Input: part model. Units: mm. Frame: model coordinates. Coordinates: 2 decimals unless noted, no trailing zeros. Order: outer loops, then holes, each group sorted by start corner. A loop starts at its lowest first (then second) coordinate and runs counter-clockwise, first axis right, second up. Notation, with made-up numbers: (-6.5, -26) -> (45.5, -26) arc R6 cw to (45.5, -19) -> close; hole circle Ø9 at (74.5, 33). An arc over 180 degrees is marked (long way). One line per question, with ' | ' between items.
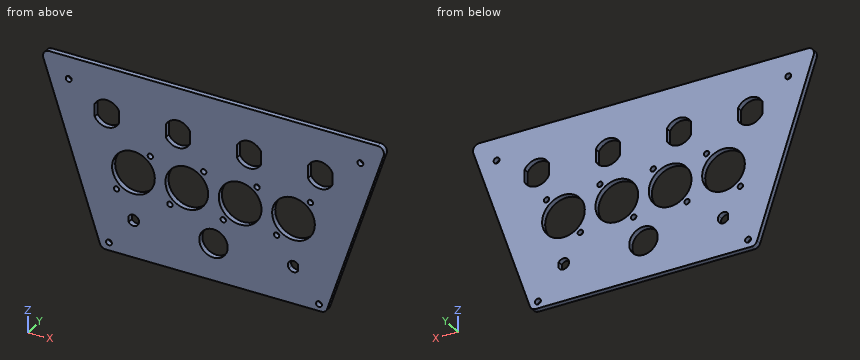
```python
from build123d import *

# Parameters (mm, degrees)
BASE_FLANGE1_DEPTH  = 3
CUT_EXTRUDE3_REACH  = 143.098
SKETCH23_R          = 12
SKETCH23_R_2        = 1.5
CUT_EXTRUDE5_REACH  = 143.098
SKETCH25_R          = 8
SKETCH30_R          = 1.65
CUT_EXTRUDE7_DEPTH  = 3
CUT_EXTRUDE9_DEPTH  = 3
CUT_EXTRUDE10_DEPTH = 3


# Sheet-metal steps are written as plain solids
with BuildPart() as part:
    # Sketch1 → Base-Flange1 (new body)
    with BuildSketch(Plane(origin=(0, 0, 0), x_dir=(1, 0, 0), z_dir=(0, 1, 0))):
        with BuildLine():
            Line((-63.892333426, 101.078420902), (-95.697333426, 5.100954406))
            ThreePointArc((-95.697333426, 5.100954406), (-95.212546513, 1.951017377), (-92.375, 0.5))
            Line((-92.375, 0.5), (92.375, 0.5))
            ThreePointArc((92.375, 0.5), (95.212546513, 1.951017377), (95.697333426, 5.100954406))
            Line((95.697333426, 5.100954406), (63.892333426, 101.078420902))
            ThreePointArc((63.892333426, 101.078420902), (62.618982623, 102.815013009), (60.57, 103.477466496))
            Line((60.57, 103.477466496), (-60.57, 103.477466496))
            ThreePointArc((-60.57, 103.477466496), (-62.618982623, 102.815013009), (-63.892333426, 101.078420902))
        make_face()
    extrude(amount=-BASE_FLANGE1_DEPTH)

    # Sketch23 → Cut-Extrude3 (cut, up to next)
    with BuildSketch(Plane(origin=(0, 0, 0), x_dir=(1, 0, 0), z_dir=(0, 1, 0)), mode=Mode.PRIVATE) as cut_extrude3_sk1:
        with Locations(Location((-45, 55.5, 0), (0, 0, 270))):
            Circle(SKETCH23_R)
    cut_extrude3_tool1 = extrude(cut_extrude3_sk1.sketch, amount=-CUT_EXTRUDE3_REACH, mode=Mode.PRIVATE) & part.part
    # Sketch23 → Cut-Extrude3 (cut, up to next)
    with BuildSketch(Plane(origin=(0, 0, 0), x_dir=(1, 0, 0), z_dir=(0, 1, 0)), mode=Mode.PRIVATE) as cut_extrude3_sk2:
        with Locations(Location((-15, 55.5, 0), (0, 0, 270))):
            Circle(SKETCH23_R)
    cut_extrude3_tool2 = extrude(cut_extrude3_sk2.sketch, amount=-CUT_EXTRUDE3_REACH, mode=Mode.PRIVATE) & part.part
    # Sketch23 → Cut-Extrude3 (cut, up to next)
    with BuildSketch(Plane(origin=(0, 0, 0), x_dir=(1, 0, 0), z_dir=(0, 1, 0)), mode=Mode.PRIVATE) as cut_extrude3_sk3:
        with Locations(Location((15, 55.5, 0), (0, 0, 270))):
            Circle(SKETCH23_R)
    cut_extrude3_tool3 = extrude(cut_extrude3_sk3.sketch, amount=-CUT_EXTRUDE3_REACH, mode=Mode.PRIVATE) & part.part
    # Sketch23 → Cut-Extrude3 (cut, up to next)
    with BuildSketch(Plane(origin=(0, 0, 0), x_dir=(1, 0, 0), z_dir=(0, 1, 0)), mode=Mode.PRIVATE) as cut_extrude3_sk4:
        with Locations(Location((45, 55.5, 0), (0, 0, 270))):
            Circle(SKETCH23_R)
    cut_extrude3_tool4 = extrude(cut_extrude3_sk4.sketch, amount=-CUT_EXTRUDE3_REACH, mode=Mode.PRIVATE) & part.part
    # Sketch23 → Cut-Extrude3 (cut, up to next)
    with BuildSketch(Plane(origin=(0, 0, 0), x_dir=(1, 0, 0), z_dir=(0, 1, 0)), mode=Mode.PRIVATE) as cut_extrude3_sk5:
        with Locations(Location((-54.5, 67.5, 0), (0, 0, 270))):
            Circle(SKETCH23_R_2)
    cut_extrude3_tool5 = extrude(cut_extrude3_sk5.sketch, amount=-CUT_EXTRUDE3_REACH, mode=Mode.PRIVATE) & part.part
    # Sketch23 → Cut-Extrude3 (cut, up to next)
    with BuildSketch(Plane(origin=(0, 0, 0), x_dir=(1, 0, 0), z_dir=(0, 1, 0)), mode=Mode.PRIVATE) as cut_extrude3_sk6:
        with Locations(Location((-35.5, 43.5, 0), (0, 0, 270))):
            Circle(SKETCH23_R_2)
    cut_extrude3_tool6 = extrude(cut_extrude3_sk6.sketch, amount=-CUT_EXTRUDE3_REACH, mode=Mode.PRIVATE) & part.part
    # Sketch23 → Cut-Extrude3 (cut, up to next)
    with BuildSketch(Plane(origin=(0, 0, 0), x_dir=(1, 0, 0), z_dir=(0, 1, 0)), mode=Mode.PRIVATE) as cut_extrude3_sk7:
        with Locations(Location((-24.5, 67.5, 0), (0, 0, 270))):
            Circle(SKETCH23_R_2)
    cut_extrude3_tool7 = extrude(cut_extrude3_sk7.sketch, amount=-CUT_EXTRUDE3_REACH, mode=Mode.PRIVATE) & part.part
    # Sketch23 → Cut-Extrude3 (cut, up to next)
    with BuildSketch(Plane(origin=(0, 0, 0), x_dir=(1, 0, 0), z_dir=(0, 1, 0)), mode=Mode.PRIVATE) as cut_extrude3_sk8:
        with Locations(Location((-5.5, 43.5, 0), (0, 0, 270))):
            Circle(SKETCH23_R_2)
    cut_extrude3_tool8 = extrude(cut_extrude3_sk8.sketch, amount=-CUT_EXTRUDE3_REACH, mode=Mode.PRIVATE) & part.part
    # Sketch23 → Cut-Extrude3 (cut, up to next)
    with BuildSketch(Plane(origin=(0, 0, 0), x_dir=(1, 0, 0), z_dir=(0, 1, 0)), mode=Mode.PRIVATE) as cut_extrude3_sk9:
        with Locations(Location((5.5, 67.5, 0), (0, 0, 270))):
            Circle(SKETCH23_R_2)
    cut_extrude3_tool9 = extrude(cut_extrude3_sk9.sketch, amount=-CUT_EXTRUDE3_REACH, mode=Mode.PRIVATE) & part.part
    # Sketch23 → Cut-Extrude3 (cut, up to next)
    with BuildSketch(Plane(origin=(0, 0, 0), x_dir=(1, 0, 0), z_dir=(0, 1, 0)), mode=Mode.PRIVATE) as cut_extrude3_sk10:
        with Locations(Location((24.5, 43.5, 0), (0, 0, 270))):
            Circle(SKETCH23_R_2)
    cut_extrude3_tool10 = extrude(cut_extrude3_sk10.sketch, amount=-CUT_EXTRUDE3_REACH, mode=Mode.PRIVATE) & part.part
    # Sketch23 → Cut-Extrude3 (cut, up to next)
    with BuildSketch(Plane(origin=(0, 0, 0), x_dir=(1, 0, 0), z_dir=(0, 1, 0)), mode=Mode.PRIVATE) as cut_extrude3_sk11:
        with Locations(Location((35.5, 67.5, 0), (0, 0, 270))):
            Circle(SKETCH23_R_2)
    cut_extrude3_tool11 = extrude(cut_extrude3_sk11.sketch, amount=-CUT_EXTRUDE3_REACH, mode=Mode.PRIVATE) & part.part
    # Sketch23 → Cut-Extrude3 (cut, up to next)
    with BuildSketch(Plane(origin=(0, 0, 0), x_dir=(1, 0, 0), z_dir=(0, 1, 0)), mode=Mode.PRIVATE) as cut_extrude3_sk12:
        with Locations(Location((54.5, 43.5, 0), (0, 0, 270))):
            Circle(SKETCH23_R_2)
    cut_extrude3_tool12 = extrude(cut_extrude3_sk12.sketch, amount=-CUT_EXTRUDE3_REACH, mode=Mode.PRIVATE) & part.part
    add(cut_extrude3_tool1.solids().sort_by_distance((-45, 0, -55.5))[0], mode=Mode.SUBTRACT)
    add(cut_extrude3_tool2.solids().sort_by_distance((-15, 0, -55.5))[0], mode=Mode.SUBTRACT)
    add(cut_extrude3_tool3.solids().sort_by_distance((15, 0, -55.5))[0], mode=Mode.SUBTRACT)
    add(cut_extrude3_tool4.solids().sort_by_distance((45, 0, -55.5))[0], mode=Mode.SUBTRACT)
    add(cut_extrude3_tool5.solids().sort_by_distance((-54.5, 0, -67.5))[0], mode=Mode.SUBTRACT)
    add(cut_extrude3_tool6.solids().sort_by_distance((-35.5, 0, -43.5))[0], mode=Mode.SUBTRACT)
    add(cut_extrude3_tool7.solids().sort_by_distance((-24.5, 0, -67.5))[0], mode=Mode.SUBTRACT)
    add(cut_extrude3_tool8.solids().sort_by_distance((-5.5, 0, -43.5))[0], mode=Mode.SUBTRACT)
    add(cut_extrude3_tool9.solids().sort_by_distance((5.5, 0, -67.5))[0], mode=Mode.SUBTRACT)
    add(cut_extrude3_tool10.solids().sort_by_distance((24.5, 0, -43.5))[0], mode=Mode.SUBTRACT)
    add(cut_extrude3_tool11.solids().sort_by_distance((35.5, 0, -67.5))[0], mode=Mode.SUBTRACT)
    add(cut_extrude3_tool12.solids().sort_by_distance((54.5, 0, -43.5))[0], mode=Mode.SUBTRACT)

    # Sketch25 → Cut-Extrude5 (cut, up to next)
    with BuildSketch(Plane(origin=(0, 0, 0), x_dir=(1, 0, 0), z_dir=(0, 1, 0)), mode=Mode.PRIVATE) as cut_extrude5_sk1:
        with Locations(Location((0, 82.5, 0), (0, 0, 270))):
            Circle(SKETCH25_R)
    cut_extrude5_tool1 = extrude(cut_extrude5_sk1.sketch, amount=-CUT_EXTRUDE5_REACH, mode=Mode.PRIVATE) & part.part
    add(cut_extrude5_tool1.solids().sort_by_distance((0, 0, -82.5))[0], mode=Mode.SUBTRACT)

    # Sketch30 → Cut-Extrude7 (cut)
    with BuildSketch(Plane.XZ.offset(3)):
        with Locations(Location((-81.400291533, -13.08225267, 0), (0, 0, 270))):
            Circle(SKETCH30_R)
        with Locations(Location((82.599708467, -13.08225267, 0), (0, 0, 270))):
            Circle(SKETCH30_R)
        with Locations(Location((-58.793005262, -98.97646978, 0), (0, 0, 270))):
            Circle(SKETCH30_R)
        with Locations(Location((59.357506456, -99.619637978, 0), (0, 0, 270))):
            Circle(SKETCH30_R)
    extrude(amount=-CUT_EXTRUDE7_DEPTH, mode=Mode.SUBTRACT)

    # Sketch32 → Cut-Extrude9 (cut)
    with BuildSketch(Plane(origin=(0, 0, 0), x_dir=(1, 0, 0), z_dir=(0, 1, 0))):
        with BuildLine():
            Line((-66.8, 30.112478374), (-66.8, 22.887521626))
            ThreePointArc((-66.8, 22.887521626), (-60, 18.8), (-53.2, 22.887521626))
            Line((-53.2, 22.887521626), (-53.2, 30.112478374))
            ThreePointArc((-53.2, 30.112478374), (-60, 34.2), (-66.8, 30.112478374))
        make_face()
        with BuildLine():
            Line((-13.2, 30.112478374), (-13.2, 22.887521626))
            ThreePointArc((-13.2, 22.887521626), (-20, 18.8), (-26.8, 22.887521626))
            Line((-26.8, 22.887521626), (-26.8, 30.112478374))
            ThreePointArc((-26.8, 30.112478374), (-20, 34.2), (-13.2, 30.112478374))
        make_face()
        with BuildLine():
            Line((26.8, 30.112478374), (26.8, 22.887521626))
            ThreePointArc((26.8, 22.887521626), (20, 18.8), (13.2, 22.887521626))
            Line((13.2, 22.887521626), (13.2, 30.112478374))
            ThreePointArc((13.2, 30.112478374), (20, 34.2), (26.8, 30.112478374))
        make_face()
        with BuildLine():
            Line((66.8, 30.112478374), (66.8, 22.887521626))
            ThreePointArc((66.8, 22.887521626), (60, 18.8), (53.2, 22.887521626))
            Line((53.2, 22.887521626), (53.2, 30.112478374))
            ThreePointArc((53.2, 30.112478374), (60, 34.2), (66.8, 30.112478374))
        make_face()
    extrude(amount=-CUT_EXTRUDE9_DEPTH, mode=Mode.SUBTRACT)

    # Sketch33 → Cut-Extrude10 (cut)
    with BuildSketch(Plane(origin=(0, 0, 0), x_dir=(1, 0, 0), z_dir=(0, 1, 0))):
        with BuildLine():
            Line((47.65, 84.202938637), (47.65, 80.797061363))
            ThreePointArc((47.65, 80.797061363), (45, 79.35), (42.35, 80.797061363))
            ThreePointArc((42.35, 80.797061363), (41.85, 82.5), (42.35, 84.202938637))
            ThreePointArc((42.35, 84.202938637), (45, 85.65), (47.65, 84.202938637))
        make_face()
    cut_extrude10 = extrude(amount=-CUT_EXTRUDE10_DEPTH, mode=Mode.SUBTRACT)

    # Mirror1: Cut-Extrude10 across plane
    add(cut_extrude10.mirror(Plane(origin=(0, 0, 0), x_dir=(0, 0, 1), z_dir=(1, 0, 0))), mode=Mode.SUBTRACT)


solid = part.part
```
1. Pin query (flat end, axial travel): pin 1 Ø14.5 at (x, z) = (-45, -55.5) entering from -Y; pin 2 Ø0.9 at (y, z) = (-1, -26) entering from -X; pin 3 Ø1.5 at (y, z) = (-2, -82) entering from +X; pin 4 Ø1 at (y, z) = (-1.5, -37) entering from +X. Return the tip coordinate at first contact, or that it passes through.
Recorded:
pin 1: passes through | pin 2: stops at x = -88.92 | pin 3: stops at x = 70.46 | pin 4: stops at x = 85.29
2. Ray query, line 1 (X direction, y = -0.9, z = -55.5); line 2 (Z direction, x = -21, y = -2.7); line 3 (X direction, y = -0.8, z = -84). Return the intervals inside material, ascending. Write a range as [from, to].
Recorded:
line 1: x = [-79, -57], [-33, -27], [-3, 3], [27, 33], [57, 79] | line 2: z = [-103.48, -65.89], [-45.11, -34.13], [-18.87, -0.5] | line 3: x = [-69.55, -47.65], [-42.23, -7.86], [7.86, 42.23], [47.65, 69.55]
3. Cut plane A-A, the plane x = 0. Return loops of the section in (y, z), and give its area (3 significant figures).
Recorded:
outline: (-3, -103.48) -> (0, -103.48) -> (0, -90.5) -> (-3, -90.5) -> close; (-3, -74.5) -> (0, -74.5) -> (0, -0.5) -> (-3, -0.5) -> close | area: 261 mm^2
4. Cut plane B-B, the plane y = -2.2. State how many separate pieces and enclosed holes the cut face has, and give its area (3 significant figures).
Recorded:
separate pieces: 1 | enclosed holes: 23 | area: 13,600 mm^2
